from build123d import *

# Parameters (mm, degrees)
F0_W      = 171.45
F0_H      = 158.75
F0_W_2    = 165.1
F0_H_2    = 152.4
F1_DEPTH  = 609.6
F3_DEPTH  = 158.751
F4_W      = 203.2
F4_H      = 284.28666
F4_W_2    = 152.4
F4_H_2    = 233.48666
F5_DEPTH  = 55.5625
F6_W      = 152.4
F6_H      = 101.6
F7_DEPTH  = 25.4
F8_W      = 160.3375
F8_H      = 4.7625
F9_DEPTH  = 4.7625
F10_W     = 160.3375
F10_H     = 4.7625
F11_DEPTH = 4.7625
F12_W     = 158.75
F12_H     = 242.466916
F13_DEPTH = 50.8


with BuildPart() as f1:
    # F0 (on Top) → F1 (new body)
    with BuildSketch(Plane.XY):
        Rectangle(F0_W, F0_H)
        Rectangle(F0_W_2, F0_H_2, mode=Mode.SUBTRACT)
    extrude(amount=F1_DEPTH)

    # F2 (on face) → F3 (cut, through all)
    with BuildSketch(Plane.XZ.offset(79.375)):
        Polygon((-85.725, 438.15), (85.725, 609.6), (-85.725, 609.6), align=None)
    extrude(amount=-F3_DEPTH, mode=Mode.SUBTRACT)

    # F4 (on face) → F5 (join)
    with BuildSketch(Plane(origin=(-261.9375, 0, 261.9375), x_dir=(0, -1, 0), z_dir=(-0.707107, 0, 0.707107))):
        with Locations((0, 370.435565)):
            Rectangle(F4_W, F4_H)
        with Locations((0, 370.435565)):
            Rectangle(F4_W_2, F4_H_2, mode=Mode.SUBTRACT)
    extrude(amount=F5_DEPTH)

    # F6 (on face) → F7 (cut)
    with BuildSketch(Plane.YZ.offset(85.725)):
        with Locations((0, 365.125)):
            Rectangle(F6_W, F6_H)
    extrude(amount=-F7_DEPTH, mode=Mode.SUBTRACT)

    # F8 (on face) → F9 (join)
    with BuildSketch(Plane(origin=(0, -76.2, 0), x_dir=(-1, 0, 0), z_dir=(0, 1, 0))):
        with Locations((2.38125, 311.94375)):
            Rectangle(F8_W, F8_H)
    extrude(amount=F9_DEPTH)

    # F10 (on face) → F11 (join)
    with BuildSketch(Plane.XZ.offset(-76.2)):
        with Locations((-2.38125, 311.94375)):
            Rectangle(F10_W, F10_H)
    extrude(amount=F11_DEPTH)

    # F12 (on face) → F13 (cut)
    with BuildSketch(Plane(origin=(-261.9375, 0, 261.9375), x_dir=(0, -1, 0), z_dir=(-0.707107, 0, 0.707107))):
        Polygon((101.6, 512.578895), (-101.6, 512.578895), (-101.6, 228.292235), (-79.375, 228.292235), (101.6, 228.292235), align=None)
        with Locations((0, 370.435565)):
            Rectangle(F12_W, F12_H, mode=Mode.SUBTRACT)
    extrude(amount=F13_DEPTH, mode=Mode.SUBTRACT)


solid = f1.part
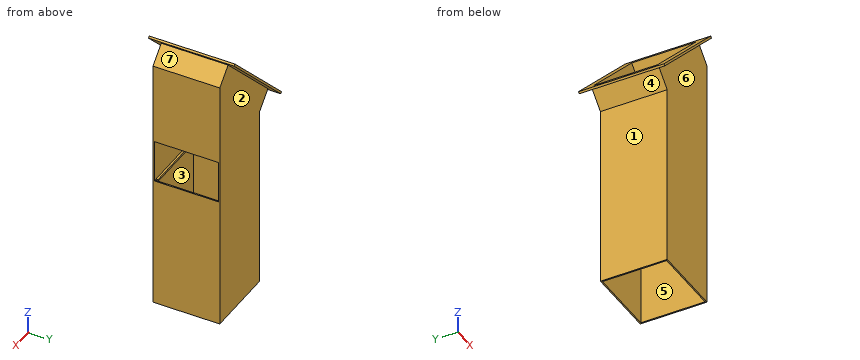
Work out the finished part from the listing and answer in its coordinate system (mm). Face numbers are marked on the shaded views. A direction names the side the tool comes from. Round coordinates to 2 decimals unless told otherwise and drop trailing zeros. Write each loop counter-clockwise with the first axis right and the second up, starting at its lowest first coordinate (ties: lowest second). Pieces come first, ordered by that corner, then holes. Notation, with made-up numbers: (81, 21.25) -> (102, 21.25) arc R29 ccw to (102, 42.25) -> close; hole circle Ø1 at (-13, 16.5). An arc over 180 degrees is marked (long way). Answer as CSV lines item,"result". Start each with the question number.
(1) The part is cut by section C-C, the plane x = -61.5. Give the vertices of the cut face in (y, z) (1 decimal), then the cut area to 3 significant figures.
(2) Find the intervals of material crossed by probe 1 along Y at (x, z) = (-10, 221) (3 decimals); probe 2 along Y at (x, z) = (57.5, 311) (1 decimal); probe 3 along X at (y, z) = (-61.5, 424.5) (3 decimals), in increasing order.
(3) The part is cut by section B-B, the plane y = -39. Give the vertices of the cut face in (x, z) (3 decimals).
(4) The part is cut by section A-A, the plane z = 427. Give the vertices of the cut face in (x, y) (3 decimals).
(5) A tool of negligible diameter and unlimited length cuts with its end or side. For the marked faces 1, 2, 3 and 4, from which of +Z, -Z, +X, -X, +Y, -Y can it reach the whole face along a straight path? Write none if from no direction.
(6) Each of these flat-tipped pins is pushed along its axis until it touches: pin 1 (3.5 mm diameter, centred on x = 84, y = -9.5, fed in from +Z) (3 decimals); pin 2 (4 mm diameter, centred on x = 22, z = 312.5, fed in from +Y) (3 decimals); pin 3 (5 mm diameter, centred on x = 27, z = 311, fed in from -Y) (3 decimals); pin 4 (4 mm diameter, centred on x = 26, y = 68.5, fed in from +Z). Where does it stop, or does it pass through?
(7) The mould has two halves that part along X. Classify the marked faces 5, 6 and 7: +X half, -X half, draft (parallel to the pull), parting line (faces both ways), or undercut.
Output values:
1,outline,"(-101.6, 534.2) -> (-79.4, 534.2) -> (-79.4, 0) -> (-76.2, 0) -> (-76.2, 309.6) -> (-71.4, 309.6) -> (-71.4, 314.3) -> (-76.2, 314.3) -> (-76.2, 541) -> (-101.6, 541) -> close; (71.4, 309.6) -> (76.2, 309.6) -> (76.2, 0) -> (79.4, 0) -> (79.4, 534.2) -> (101.6, 534.2) -> (101.6, 541) -> (76.2, 541) -> (76.2, 314.3) -> (71.4, 314.3) -> close"
1,area,"3,780 mm²"
2,probe 1,"y = -79.375 to -76.2, 76.2 to 79.375"
2,probe 2,"y = -79.4 to -71.4, 71.4 to 79.4"
2,probe 3,"x = -85.725 to -82.55, 82.55 to 85.725"
3,outline,"(-139.799, 462.653) -> (-136.432, 459.286) -> (-121.646, 474.071) -> (-85.725, 438.15) -> (-85.725, 0) -> (-82.55, 0) -> (-82.55, 441.325) -> (-121.839, 480.614) -> close; (43.261, 645.714) -> (82.55, 606.425) -> (82.55, 415.925) -> (85.725, 415.925) -> (85.725, 609.6) -> (49.804, 645.521) -> (64.589, 660.307) -> (61.222, 663.674) -> close; (82.55, 0) -> (85.725, 0) -> (85.725, 314.325) -> (82.55, 314.325) -> close"
4,outline,"(-85.725, -79.375) -> (85.725, -79.375) -> (85.725, 79.375) -> (-85.725, 79.375) -> close; hole (-82.55, -76.2) -> (82.55, -76.2) -> (82.55, 76.2) -> (-82.55, 76.2) -> close"
5,face 1,"-Z, -X, +Y, -Y"
5,face 2,"-Z, +X, +Y"
5,face 3,"none"
5,face 4,"-Z, +Y, -Y"
6,pin 1,"stops at z = 613.075"
6,pin 2,"stops at y = 79.375"
6,pin 3,"stops at y = -79.375"
6,pin 4,"passes through"
7,face 5,"undercut"
7,face 6,"draft"
7,face 7,"+X half"
